Model file for the job. Use its own axes, mm. Face numbers are marked on the shaded views. Round coordinates to 2 decimals unless told otherwise and drop trailing zeros. Order: outer loops, then holes, each group sorted by start corner. A loop starts at its lowest first (then second) coordinate and runs counter-clockwise, first axis right, second up. Notation, with made-up numbers: (72.25, 76) - (83.25, 76) arc R33 ccw to (83.25, 112) - close; hole circle Ø5 at (80, -9). An arc over 180 degrees is marked (long way). Answer as CSV lines item,"result". Start each with the question number.
1. Wall check: line 1 along X through (y, z) = (0, -3); line 2 along X through (y, z) = (2.5, -0.9); line 3 along Y through (x, z) = (3.25, -3.85). Give the ranges that are in metal, low to high. Write a range as [from, to].
2. Band-saw the part on A-A on z = -3.9. List the corners of the cut face in (x, y).
3. Pull direction Y, two halves, no side cores. Call the marked faces 1, 2, 3 and 4: released by +Y, released by -Y, zero draft, split by the parting line, or undercut.
4. Pin check, flat tips, straight feed: pin 1 Ø6 at (x, y) = (-0.5, -1.5) entering from +Z; pin 2 Ø3 at (x, z) = (2, -1) entering from +Y. Stop position of each tip, or through.
```python
from build123d import *

# Parameters (mm, degrees)
SKETCH2_W          = 28.448
SKETCH2_H          = 28.448
CUT_EXTRUDE1_DEPTH = 5.588


with BuildPart() as part:
    # Sketch1 → Revolve1 (revolve)
    with BuildSketch(Plane(origin=(0, 0, 0), x_dir=(0, 0, -1), z_dir=(1, 0, 0))):
        Polygon((0, 0), (0, 7.112), (0.381130931, 8.5344), (5.206869069, 8.5344), (5.588, 7.112), (5.588, 0), align=None)
    revolve(axis=Axis((0, 0, -5.588), (0, 0, 1)))

    # Sketch2 → Cut-Extrude1 (cut)
    with BuildSketch(Plane.XY):
        Rectangle(SKETCH2_W, SKETCH2_H)
        Polygon((-7.112, -4.106115114), (0, -8.212230229), (7.112, -4.106115114), (7.112, 4.106115114), (0, 8.212230229), (-7.112, 4.106115114), align=None, mode=Mode.SUBTRACT)
    extrude(amount=-CUT_EXTRUDE1_DEPTH, mode=Mode.SUBTRACT)

    # Sketch3 → Cut-Revolve1 (revolve, cut)
    with BuildSketch(Plane(origin=(0, 0, 0), x_dir=(0, 0, -1), z_dir=(1, 0, 0))):
        Polygon((0, 0), (0, 4.7625), (0.57277, 4.18973), (5.01523, 4.18973), (5.588, 4.7625), (5.588, 0), align=None)
    revolve(axis=Axis((0, 0, -5.588), (0, 0, 1)), mode=Mode.SUBTRACT)


solid = part.part
```
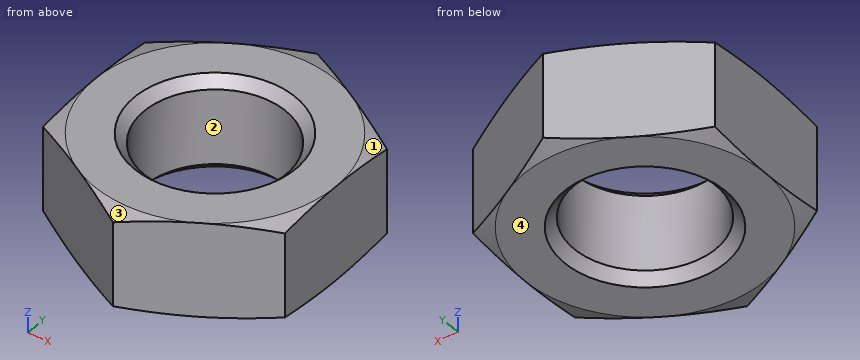
Reply:
1,line 1,"x = [-7.11, -4.19], [4.19, 7.11]"
1,line 2,"x = [-7.11, -3.36], [3.36, 7.11]"
1,line 3,"y = [-6.34, -2.64], [2.64, 6.34]"
2,outline,"(-7.11, -4.11) - (0, -8.21) - (7.11, -4.11) - (7.11, 4.11) - (0, 8.21) - (-7.11, 4.11) - close; hole circle Ø8.38 at (0, 0)"
3,face 1,"released by +Y"
3,face 2,"undercut"
3,face 3,"released by -Y"
3,face 4,"zero draft"
4,pin 1,"stops at z = -0.18"
4,pin 2,"stops at y = 7.92"
